Input: part model. Units: mm. Frame: model coordinates. A direction names the side the tool comes from. Coordinates: 2 decimals unless noted, no trailing zeros. Order: outer loops, then holes, each group sorted by start corner. A loop starts at its lowest first (then second) coordinate and runs counter-clockwise, first axis right, second up. Notation, with made-up numbers: (23, -7) -> (30, -7) arc R5 cw to (30, -3) -> close; hole circle Ø7 at (43, 7.5). An arc over 180 degrees is marked (long way). Write each question's results on one line, items separated by ' | '.
```python
from build123d import *

# Parameters (mm, degrees)
F0_R          = 0.8
F1_DEPTH      = 13
F2_R          = 6.25
F3_DEPTH      = 1
F3_DEPTH_BACK = 27
F4_R          = 3
F4_R_2        = 1.5
F5_DEPTH      = 3.5
F6_R          = 3.5
F6_R_2        = 1.1
F7_DEPTH      = 2
F8_W          = 13.45
F8_H          = 6.1
F9_DEPTH      = 5


with BuildPart() as f1:
    # F0 (on Top) → F1 (new body, symmetric)
    with BuildSketch(Plane.XY):
        with BuildLine():
            Line((-23.5, 10.5), (-23.5, 0))
            Line((-23.5, 0), (-23.5, -10.5))
            ThreePointArc((-23.5, -10.5), (-22.767767, -12.267767), (-21, -13))
            Line((-21, -13), (0, -13))
            ThreePointArc((0, -13), (4.25883, -12.282604), (8.047619, -10.209595))
            ThreePointArc((8.047619, -10.209595), (8.749339, -9.337301), (9, -8.246211))
            Line((9, -8.246211), (9, 0))
            Line((9, 0), (9, 8.246211))
            ThreePointArc((9, 8.246211), (8.749339, 9.337301), (8.047619, 10.209595))
            ThreePointArc((8.047619, 10.209595), (4.25883, 12.282604), (0, 13))
            Line((0, 13), (-21, 13))
            ThreePointArc((-21, 13), (-22.767767, 12.267767), (-23.5, 10.5))
        make_face()
        with Locations((-21, -10.5)):
            Circle(F0_R, mode=Mode.SUBTRACT)
        with Locations((0, -10.5)):
            Circle(F0_R, mode=Mode.SUBTRACT)
        with Locations((-21, 10.5)):
            Circle(F0_R, mode=Mode.SUBTRACT)
        with Locations((0, 10.5)):
            Circle(F0_R, mode=Mode.SUBTRACT)
    extrude(amount=F1_DEPTH, both=True)

    # F2 (on face) → F3 (join, two sides)
    with BuildSketch(Plane.XY.offset(13)) as f3_sk:
        Circle(F2_R)
    extrude(amount=F3_DEPTH)
    extrude(f3_sk.sketch, amount=-F3_DEPTH_BACK)

    # F4 (on face) → F5 (join)
    with BuildSketch(Plane.XY.offset(14)):
        Circle(F4_R)
        Circle(F4_R_2, mode=Mode.SUBTRACT)
    extrude(amount=F5_DEPTH)

    # F6 (on face) → F7 (join)
    with BuildSketch(Plane(origin=(0, 0, -14), x_dir=(1, 0, 0), z_dir=(0, 0, -1))):
        Circle(F6_R)
        Circle(F6_R_2, mode=Mode.SUBTRACT)
    extrude(amount=F7_DEPTH)

    # F8 (on face) → F9 (join)
    with BuildSketch(Plane.XZ.offset(13)):
        with Locations((-10.725, -6.85)):
            Rectangle(F8_W, F8_H)
    extrude(amount=F9_DEPTH)


solid = f1.part
```
(1) Cut plane A-A, the plane z = 10. Return loops of the section in (x, y).
Return value:
outline: (-23.5, -10.5) arc R2.5 ccw to (-21, -13) -> (0, -13) arc R13 ccw to (8.05, -10.21) arc R2.5 ccw to (9, -8.25) -> (9, 8.25) arc R2.5 ccw to (8.05, 10.21) arc R13 ccw to (0, 13) -> (-21, 13) arc R2.5 ccw to (-23.5, 10.5) -> close; hole circle Ø1.6 at (-21, -10.5); hole circle Ø1.6 at (-21, 10.5); hole circle Ø1.6 at (0, -10.5); hole circle Ø1.6 at (0, 10.5)
(2) Pin query (flat end, axial travel): P1, Ø0.9, axis at x = 0.5, y = 0.5, coming from the +Z side; P2, Ø4, axis at y = -14.5, z = -6.5, coming from the -X side; P3, Ø0.7, axis at x = -0.5, y = 0, coming from the -Z side; P4, Ø1.4, axis at x = 0, y = 10.5, coming from the +Z side. Return the tip coordinate at first contact, or that it passes through.
Return value:
P1: z = 14 | P2: x = -22.5 | P3: z = -14 | P4: through
(3) Cut plane D-D, the plane z = -7.5. Return loops of the section in (x, y).
Return value:
outline: (-23.5, -10.5) arc R2.5 ccw to (-21, -13) -> (-17.45, -13) -> (-17.45, -18) -> (-4, -18) -> (-4, -13) -> (0, -13) arc R13 ccw to (8.05, -10.21) arc R2.5 ccw to (9, -8.25) -> (9, 8.25) arc R2.5 ccw to (8.05, 10.21) arc R13 ccw to (0, 13) -> (-21, 13) arc R2.5 ccw to (-23.5, 10.5) -> close; hole circle Ø1.6 at (-21, -10.5); hole circle Ø1.6 at (-21, 10.5); hole circle Ø1.6 at (0, -10.5); hole circle Ø1.6 at (0, 10.5)
(4) Cut plane B-B, the plane y = 0. Return loops of the section in (x, z), plus the area to 3 significant figures.
Return value:
outline: (-23.5, -13) -> (-6.25, -13) -> (-6.25, -14) -> (-3.5, -14) -> (-3.5, -16) -> (-1.1, -16) -> (-1.1, -14) -> (1.1, -14) -> (1.1, -16) -> (3.5, -16) -> (3.5, -14) -> (6.25, -14) -> (6.25, -13) -> (9, -13) -> (9, 13) -> (6.25, 13) -> (6.25, 14) -> (3, 14) -> (3, 17.5) -> (1.5, 17.5) -> (1.5, 14) -> (-1.5, 14) -> (-1.5, 17.5) -> (-3, 17.5) -> (-3, 14) -> (-6.25, 14) -> (-6.25, 13) -> (-23.5, 13) -> close | area: 890 mm2
(5) Reachability of faces 1 (the face through (0, 0, -14)), 2 (the face through (-3, 0, 16)), 3 (the face through (-17.45, -15, -7)), 4 (the face through (-21.104, -9.707, -0.182)), 5 (the face through (9, 0, 0)) from +Z, -Z, +X, -X, +Y, -Y: full face, straight path, thin tool, end or side. Return the list, or none.
Return value:
face 1: -Z | face 2: +Z | face 3: +Z, -Z, -X, -Y | face 4: +Z, -Z | face 5: +Z, -Z, +X, +Y, -Y
(6) Line query: line 1 along Y through (x, z) = (-21, 0); line 2 along Z through (x, y) = (-13.5, -7); line 3 along Y through (x, z) = (0, -15.2). Output: solid intervals per line, ascending. Write a range as from..to.
Return value:
line 1: -13..-11.3, -9.7..9.7, 11.3..13 | line 2: -13..13 | line 3: -3.5..-1.1, 1.1..3.5
(7) Mould query, pull axis Y, two halves, no side actions, for faces 6 (the face through (1.05, -0.33, -14.99)), 7 (the face through (3.233, 1.341, -14.986)), 8 (the face through (-23.5, 0, 0)). Classes: +Y half, -Y half, draft (parallel to the pull), parting line (faces both ways), or undercut.
Return value:
face 6: undercut | face 7: parting line | face 8: draft
(8) Cut plane C-C, the plane x = -14. Return loops of the section in (y, z).
Return value:
outline: (-18, -9.9) -> (-13, -9.9) -> (-13, -13) -> (13, -13) -> (13, 13) -> (-13, 13) -> (-13, -3.8) -> (-18, -3.8) -> close
